Source: CAD feature listing. Evaluate the final solid. Frame: model axes, mm. A direction names the side the tool comes from. Give positions to 0.01 mm unless a question says otherwise; leave off trailing zeros. Order: outer loops, then holes, each group sorted by start corner. A loop starts at its lowest first (then second) coordinate and runs counter-clockwise, first axis right, second up. Notation, with made-up numbers: (76, 42) -> (89, 42) arc R37 cw to (89, 80) -> close; hole circle Ø6 at (-13.5, 61). An arc over 180 degrees is marked (long way). Use CSV: the item, a comma, the result in double quotes.
```python
from build123d import *

# Parameters (mm, degrees)
F0_R     = 26.67
F1_DEPTH = 67.7418
F2_W     = 22.225
F2_H     = 22.225
F3_DEPTH = 67.7418
F4_R     = 11.11249
F5_R     = 1.7272
F6_DEPTH = 5.5800505253


# Not quite as in the source:
# - a fillet or chamfer is up to 0.001 mm smaller than in the source, because OpenCascade refuses the exact size


with BuildPart() as f1:
    # F0 (on Top) → F1 (new body)
    with BuildSketch(Plane.XY):
        Circle(F0_R)
    extrude(amount=F1_DEPTH)

    # F2 (on face) → F3 (cut, through all)
    with BuildSketch(Plane.XY.offset(67.7418)):
        with Locations((0, -15.5575)):
            Rectangle(F2_W, F2_H)
    extrude(amount=-F3_DEPTH, mode=Mode.SUBTRACT)

    # F4 (radius 11.1125 in the source; OpenCascade refuses exactly that, so slightly less here)
    f4_edges = [f1.edges().sort_by_distance(p)[0] for p in [
        (11.1125, -4.445, 33.8709),
        (-11.1125, -4.445, 33.8709),
    ]]
    fillet(f4_edges, radius=F4_R)

    # F5 (on Front) → F6 (cut, up to face)
    with BuildSketch(Plane.XZ):
        with Locations((0, 33.8709)):
            Circle(F5_R)
    extrude(amount=F6_DEPTH, mode=Mode.SUBTRACT)


solid = f1.part
```
1. Section query C-C on y = -5.5. Return loops of the section in (x, z).
Answer below:
outline,"(-26.1, 0) -> (-4.73, 0) -> (-4.73, 67.74) -> (-26.1, 67.74) -> close; (4.73, 0) -> (26.1, 0) -> (26.1, 67.74) -> (4.73, 67.74) -> close"
2. Pin query (flat end, axial travel): P1, Ø5.5, axis at x = 0, z = 33.87, coming from the +Y side; P2, Ø9.5, axis at y = -22, z = 30.5, coming from the -X side; P3, Ø2, axis at y = 16, z = 19, coming from the -X side. Return the tip coordinate at first contact, or that it passes through.
Answer below:
P1,"stops at y = 26.67"
P2,"stops at x = -20.34"
P3,"stops at x = -22.05"
3. Section query A-A on y = -18. Return loops of the section in (x, z), plus the area to 3 significant figures.
Answer below:
outline,"(-19.68, 0) -> (-11.11, 0) -> (-11.11, 67.74) -> (-19.68, 67.74) -> close; (11.11, 0) -> (19.68, 0) -> (19.68, 67.74) -> (11.11, 67.74) -> close"
area,"1,160 mm²"
4. Access query for faces 1 (the cylindrical face through (-0.374, -2.258, 32.185)), 2 (the cylindrical face through (7.771, -7.614, 33.397)), 3 (the cylindrical face through (1.01, 26.65, 33.4)). Directions: +Z, -Z, +X, -X, +Y, -Y. A direction counts if a zero-diameter tool reaches every point of the face in a straight line with its end or side. Return the directions, or none.
Answer below:
face 1,"-Y"
face 2,"+Z, -Z, -Y"
face 3,"+Z, -Z"
5. Mould query, pull axis Z, two halves, no side actions, for faces 4 (the flat face through (0, 2, 67.742)), 5 (the flat face through (0, 0, 34)), 6 (the cylindrical face through (-7.944, -7.787, 33.397)). Classes: released by +Z, released by -Z, zero draft, split by the parting line, or undercut.
Answer below:
face 4,"released by +Z"
face 5,"undercut"
face 6,"zero draft"
6. Section query D-D on x = 12. Return loops of the section in (y, z), plus the area to 3 significant figures.
Answer below:
outline,"(-23.82, 0) -> (23.82, 0) -> (23.82, 67.74) -> (-23.82, 67.74) -> close"
area,"3,230 mm²"
7. Section query B-B on z = 33. Return loops of the section in (x, y), plus the area to 3 significant figures.
Answer below:
outline,"(-11.11, -24.24) -> (-11.11, -15.56) arc R11.11 cw to (-1.49, -4.55) -> (-1.49, 0) -> (1.49, 0) -> (1.49, -4.55) arc R11.11 cw to (11.11, -15.56) -> (11.11, -24.24) arc R26.67 ccw (long way) to start"
area,"1,800 mm²"
8. Ray query, line 1 along Z through (x, y) = (0, -1); line 2 along X through (y, z) = (-16, 5.5); line 3 along X through (y, z) = (-18.5, 20). Return the intervals inside material, ascending.
Answer below:
line 1,"z = 0 to 32.14, 35.6 to 67.74"
line 2,"x = -21.34 to -11.11, 11.11 to 21.34"
line 3,"x = -19.21 to -11.11, 11.11 to 19.21"
